Read the model definition and answer for the solid it produces. Units are mm, in the model's axes. Face numbers are marked on the shaded views. A direction names the side the tool comes from. Round coordinates to 2 decimals unless told otherwise and drop trailing zeros. Order: outer loops, then holes, each group sorted by start corner. A loop starts at its lowest first (then second) coordinate and runs counter-clockwise, first axis right, second up.
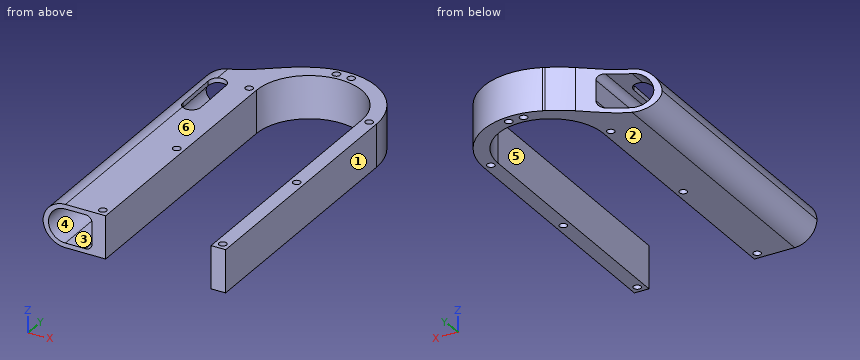
from build123d import *

# Parameters (mm, degrees)
BOSS_EXTRUDE1_DEPTH = 19.05
SKETCH2_R           = 1.7
CUT_EXTRUDE1_DEPTH  = 302.810637772
CUT_EXTRUDE2_DEPTH  = 302.810637772
BOSS_EXTRUDE2_DEPTH = 135
BOSS_EXTRUDE3_START = -19.05
BOSS_EXTRUDE3_DEPTH = 19.05
CUT_EXTRUDE4_DEPTH  = 316.043777756
CUT_EXTRUDE5_DEPTH  = 249.524391307
CUT_EXTRUDE6_DEPTH  = 7
FILLET1_R           = 50
FILLET2_R           = 10
FILLET3_R           = 3


with BuildPart() as part:
    # Sketch1 → Boss-Extrude1 (new body)
    with BuildSketch(Plane.XY):
        with BuildLine():
            Line((-179.085368151, -18.789194183), (-179.085368151, 212.188334746))
            ThreePointArc((-179.085368151, 212.188334746), (-149.085368151, 242.188334746), (-119.085368151, 212.188334746))
            Line((-119.085368151, 212.188334746), (-119.085368151, -18.789194183))
            ThreePointArc((-119.085368151, -18.789194183), (-149.085368151, -48.789194183), (-179.085368151, -18.789194183))
        make_face()
        with BuildLine():
            Line((-172.585368151, -18.789194183), (-172.585368151, 212.188334746))
            ThreePointArc((-172.585368151, 212.188334746), (-149.085368151, 235.688334746), (-125.585368151, 212.188334746))
            Line((-125.585368151, 212.188334746), (-125.585368151, -18.789194183))
            ThreePointArc((-125.585368151, -18.789194183), (-149.085368151, -42.289194183), (-172.585368151, -18.789194183))
        make_face(mode=Mode.SUBTRACT)
    extrude(amount=BOSS_EXTRUDE1_DEPTH)

    # Sketch2 → Cut-Extrude1 (cut, through all)
    with BuildSketch(Plane.XY.offset(19.05)):
        with Locations((-145.785368151, 238.734002942)):
            Circle(SKETCH2_R)
        with Locations((-122.335368151, 212.188334746)):
            Circle(SKETCH2_R)
        with Locations((-152.485368151, -45.322239617)):
            Circle(SKETCH2_R)
        with Locations((-168.000474547, -37.70430058)):
            Circle(SKETCH2_R)
        with Locations((-175.835368151, -18.789194183)):
            Circle(SKETCH2_R)
        with Locations((-175.835368151, 212.188334746)):
            Circle(SKETCH2_R)
        with Locations((-145.685368151, -45.322239617)):
            Circle(SKETCH2_R)
        with Locations((-175.835368151, 100.099570281)):
            Circle(SKETCH2_R)
        with Locations((-175.835368151, 93.299570281)):
            Circle(SKETCH2_R)
        with Locations((-122.335368151, 100.099570281)):
            Circle(SKETCH2_R)
        with Locations((-122.335368151, 93.299570281)):
            Circle(SKETCH2_R)
        with Locations((-122.335368151, -18.789194183)):
            Circle(SKETCH2_R)
        with Locations((-130.170261754, -37.70430058)):
            Circle(SKETCH2_R)
        with Locations((-175.835368151, 156.699570281)):
            Circle(SKETCH2_R)
        with Locations((-122.335368151, 156.699570281)):
            Circle(SKETCH2_R)
        with Locations((-175.835368151, 66.699570281)):
            Circle(SKETCH2_R)
        with Locations((-122.335368151, 66.699570281)):
            Circle(SKETCH2_R)
        with Locations((-175.835368151, 36.699570281)):
            Circle(SKETCH2_R)
        with Locations((-122.335368151, 36.699570281)):
            Circle(SKETCH2_R)
        with Locations((-175.835368151, 6.699570281)):
            Circle(SKETCH2_R)
        with Locations((-122.335368151, 6.699570281)):
            Circle(SKETCH2_R)
        with Locations((-152.385368151, 238.734002942)):
            Circle(SKETCH2_R)
    extrude(amount=-CUT_EXTRUDE1_DEPTH, mode=Mode.SUBTRACT)

    # Sketch3 → Cut-Extrude2 (cut, through all)
    with BuildSketch(Plane.XY.offset(19.05)):
        Polygon((-149.085368151, 96.699570281), (-100.167336626, 96.699570281), (-100.167336626, -59.171887956), (-212.527814826, -59.171887956), (-212.527814826, 96.699570281), align=None)
    extrude(amount=-CUT_EXTRUDE2_DEPTH, mode=Mode.SUBTRACT)

    # Sketch4 → Boss-Extrude2 (add)
    with BuildSketch(Plane.XZ.offset(-96.699570281)):
        with BuildLine():
            Line((-179.085368151, 19.05), (-196.652205402, 19.05))
            ThreePointArc((-196.652205402, 19.05), (-200.585368151, 9.525), (-196.652205402, 0))
            Line((-196.652205402, 0), (-179.085368151, 0))
            Line((-179.085368151, 0), (-179.085368151, 19.05))
        make_face()
    extrude(amount=-BOSS_EXTRUDE2_DEPTH)

    # Sketch5 → Boss-Extrude3 (add)
    with BuildSketch(Plane.XY.offset(19.05).offset(BOSS_EXTRUDE3_START)):
        with BuildLine():
            Line((-179.085368151, 231.699570281), (-179.085368151, 212.188334746))
            ThreePointArc((-179.085368151, 212.188334746), (-174.234371945, 228.544605963), (-161.250194275, 239.611263206))
            Line((-161.250194275, 239.611263206), (-179.085368151, 231.699570281))
        make_face()
    extrude(amount=BOSS_EXTRUDE3_DEPTH)

    # Sketch6 → Cut-Extrude4 (cut, through all)
    with BuildSketch(Plane.XY.offset(19.05)):
        with BuildLine():
            Line((-166.948269283, 237.083594004), (-200.585368151, 237.083594004))
            Line((-200.585368151, 237.083594004), (-200.585368151, 215.169829532))
            add(Edge.make_bspline(
                [(-166.948269283, 237.083594004), (-174.08025285, 232.264666523), (-185.619403498, 221.256742546), (-196.521569709, 219.674382376), (-200.585368151, 215.169829532)],
                knots=[0, 0, 0, 0, 0.58548773, 1, 1, 1, 1], degree=3))
        make_face()
    extrude(amount=-CUT_EXTRUDE4_DEPTH, mode=Mode.SUBTRACT)

    # Sketch7 → Cut-Extrude5 (cut, through all)
    with BuildSketch(Plane.XZ.offset(-96.699570281)):
        with BuildLine():
            Line((-190.585368151, 17.025), (-178.585368151, 17.025))
            Line((-178.585368151, 17.025), (-178.585368151, 2.025))
            Line((-178.585368151, 2.025), (-190.585368151, 2.025))
            ThreePointArc((-190.585368151, 2.025), (-198.085368151, 9.525), (-190.585368151, 17.025))
        make_face()
    extrude(amount=-CUT_EXTRUDE5_DEPTH, mode=Mode.SUBTRACT)

    # Sketch8 → Cut-Extrude6 (cut)
    with BuildSketch(Plane.XY.offset(19.05)):
        with BuildLine():
            Line((-184.578582607, 209.622626451), (-184.241218911, 189.62547201))
            ThreePointArc((-184.241218911, 189.62547201), (-188.17317706, 185.558568382), (-192.240080687, 189.490526531))
            Line((-192.240080687, 189.490526531), (-192.577444383, 209.487680972))
            ThreePointArc((-192.577444383, 209.487680972), (-188.645486234, 213.554584599), (-184.578582607, 209.622626451))
        make_face()
    extrude(amount=-CUT_EXTRUDE6_DEPTH, mode=Mode.SUBTRACT)

    # Fillet1
    fillet1_edges = [part.edges().sort_by_distance(p)[0] for p in [
        (-166.948269283, 237.083594004, 9.525),
    ]]
    fillet(fillet1_edges, radius=FILLET1_R)

    # Fillet2
    # the kernel refuses this fillet: 10 mm, written as the material it takes off along each edge
    with BuildSketch(Plane(origin=(-196.652205402, 66.752998532, 0), x_dir=(1, 0, 0), z_dir=(0, 1, 0))) as fillet2_piece_1:
        with BuildLine():
            CenterArc((6.099219193, -10), FILLET2_R, 90, 97.799925588)
            ThreePointArc((-3.808260974, -11.357142857), (-3.23274377, -5.233062714), (0, 0))
            Line((0, 0), (6.099219193, 0))
        make_face()
    extrude(amount=181.626081549, mode=Mode.SUBTRACT)
    with BuildSketch(Plane(origin=(-196.652205402, 66.752998532, 19.05), x_dir=(-0.3179212804444137, 0, -0.9481171127242586), z_dir=(0, 1, 0))) as fillet2_piece_2:
        with BuildLine():
            CenterArc((7.542099552, -8.961986896), FILLET2_R, 63.66281519, 97.799925588)
            Line((-1.939071576, -5.782774091), (0, 0))
            ThreePointArc((0, 0), (5.98931435, 1.401317691), (11.9786287, 0))
        make_face()
    extrude(amount=181.626081549, mode=Mode.SUBTRACT)

    # Fillet3
    fillet3_edges = [part.edges().sort_by_distance(p)[0] for p in [
        (-178.585368151, 162.512316203, 17.025),
        (-178.585368151, 162.512316203, 2.025),
    ]]
    fillet(fillet3_edges, radius=FILLET3_R)


solid = part.part
Q1. For the marked faces 4, 5 and 6, determine the directions among +Z, -Z, +X, -X, +Y, -Y from which every point of the face is accessible in a straight line to the end or side of a thin tool.
Outcome:
face 4: +Y, -Y
face 5: +Z, -Z, -Y
face 6: +Z, +X, -X, +Y, -Y
Q2. A cutting plane is placed at A-A, the plane y = 113. Give the vertices of the cut face in (x, z) (3 decimals).
Outcome:
outline: (-200.542, 9.525) arc R10 ccw to (-190.553, 0) - (-172.585, 0) - (-172.585, 19.05) - (-190.553, 19.05) arc R10 ccw to start; (-125.585, 0) - (-119.085, 0) - (-119.085, 19.05) - (-125.585, 19.05) - close; hole (-190.585, 2.025) - (-181.585, 2.025) arc R3 ccw to (-178.585, 5.025) - (-178.585, 14.025) arc R3 ccw to (-181.585, 17.025) - (-190.585, 17.025) arc R7.5 ccw to start
Q3. A cutting plane is placed at C-C, the plane z = 12.5. Give the number of separate pieces and of enclosed holes in the cut face, plus the area to 3 significant figures.
Outcome:
separate pieces: 2
enclosed holes: 8
area: 2,250 mm2
Q4. Straight lines are drawn through the part: probe 1 along X at (y, z) = (132, 11); probe 2 along X at (y, z) = (103.5, 4.25); probe 3 along Z at (x, y) = (-186.5, 216.5) (3 decimals). For each, find the intervals that lie inside material, in ascending order.
Outcome:
probe 1: x = -200.36 to -197.94, -178.59 to -172.59, -125.59 to -119.09
probe 2: x = -198.73 to -195.92, -178.69 to -172.59, -125.59 to -119.09
probe 3: z = 0 to 2.025, 17.025 to 19.05
Q5. Flat-ended cylindrical pins translate along their axes: pin 1 (10 mm diameter, centred on x = -169, y = 218.5, fed in from -Z); pin 2 (10 mm diameter, centred on x = -135.5, z = 3.5, fed in from +Y); pin 3 (1 mm diameter, centred on x = -177, z = 14.5, fed in from +Y). Find the tip coordinate at first contact, or state that the pin passes through.
Outcome:
pin 1: stops at z = 0
pin 2: stops at y = 240.93
pin 3: stops at y = 229.93
Q6. A cutting plane is placed at D-D, the plane x = -131. Give the vertices of the cut face in (y, z).
Outcome:
outline: (227.19, 0) - (236.12, 0) - (236.12, 19.05) - (227.19, 19.05) - close
Q7. For a pull along X with two mould halves and no side action, classify the marked faces 1, 2 and 3 as released by +X, released by -X, zero draft, split by the parting line, or undercut.
Outcome:
face 1: released by +X
face 2: zero draft
face 3: undercut
Q8. A cutting plane is placed at B-B, the plane y = 206. Give the vertices of the cut face in (x, z) (3 decimals).
Outcome:
outline: (-200.542, 9.525) arc R10 ccw to (-190.553, 0) - (-172.585, 0) - (-172.585, 19.05) - (-184.517, 19.05) - (-184.517, 17.025) - (-181.585, 17.025) arc R3 cw to (-178.585, 14.025) - (-178.585, 5.025) arc R3 cw to (-181.585, 2.025) - (-190.585, 2.025) arc R7.5 cw to (-192.519, 16.772) - (-192.519, 18.855) arc R10 ccw to start; (-125.585, 0) - (-119.085, 0) - (-119.085, 19.05) - (-125.585, 19.05) - close
